The model under review builds one solid part; all positions refer to its coordinate system, in mm. A direction names the side the tool comes from. Round coordinates to 2 decimals unless told otherwise and drop trailing zeros. Write each loop counter-clockwise with the first axis right and the second up, starting at its lowest first coordinate (ties: lowest second). Pieces come first, ordered by that corner, then holes.
Item 1: Clearance check with flat-ended pins moving along their axes: pin 1 Ø5 at (y, z) = (-52, -5) entering from -X; pin 2 Ø8 at (x, y) = (-6.5, 62) entering from -Z; pin 3 Ø3 at (x, y) = (-4.5, 1) entering from +Z. State where each tip first meets the part, or that it passes through.
Item 2: Add section A-A (x = 0). Give the boundary of the cut face in (y, z) (3 decimals).
Item 3: Add section D-D (y = -61.5). Give the boundary of the cut face in (x, z) (3 decimals).
Item 4: Add section B-B (z = 0). Give the boundary of the cut face in (x, y) (3 decimals).
Item 5: Draft analysis for pull direction X (two halves, no side actions). For faces 1 (the face through (-7.559, -1.378, -5.796)), 2 (the face through (0, -66.675, 0)), 3 (the face through (0, 66.675, 0)), 4 (the face through (4, 98.425, -4)), state which applies: +X half, -X half, draft (parallel to the pull), parting line (faces both ways), or undercut.
Item 6: Add section C-C (y = 75.5). Give the boundary of the cut face in (x, z) (3 decimals), plus the area to 3 significant figures.
Item 7: Machinability: for faces 5 (the face through (0, -98.425, -6)), 6 (the face through (5.49, -82.77, 1.73)), 7 (the face through (-4.73, 82.77, 1.49)), which of the approach directions +Z, -Z, +X, -X, +Y, -Y give a long, thin tool a straight path to every point of the face, cutting with its end or side? Answer none if there is none.
Item 8: To check wall thickness, follow L1, parallel to Z at x = -0.25, y = 71; L2, parallel to Z at x = 0, y = -77 (3 decimals); L3, parallel to Y at x = 4.25, z = 3.25 (3 decimals). State the ranges of each line that lie inside material, in increasing order.
```python
from build123d import *

# Parameters (mm, degrees)
F0_R     = 9.525
F1_DEPTH = 98.425
F2_R     = 5.754688
F3_DEPTH = 31.75
F4_R     = 4.960938
F5_DEPTH = 31.75


with BuildPart() as f1:
    # F0 (on Front) → F1 (new body, symmetric)
    with BuildSketch(Plane.XZ):
        Circle(F0_R)
    extrude(amount=F1_DEPTH, both=True)

    # F2 (on face) → F3 (cut)
    with BuildSketch(Plane.XZ.offset(98.425)):
        Circle(F2_R)
    extrude(amount=-F3_DEPTH, mode=Mode.SUBTRACT)

    # F4 (on face) → F5 (cut)
    with BuildSketch(Plane(origin=(0, 98.425, 0), x_dir=(-1, 0, 0), z_dir=(0, 1, 0))):
        Circle(F4_R)
    extrude(amount=-F5_DEPTH, mode=Mode.SUBTRACT)


solid = f1.part
```
Numbers:
1. pin 1: stops at x = -9.19
1. pin 2: stops at z = -9.19
1. pin 3: stops at z = 9.04
2. outline: (-98.425, -9.525) - (98.425, -9.525) - (98.425, -4.961) - (66.675, -4.961) - (66.675, 4.961) - (98.425, 4.961) - (98.425, 9.525) - (-98.425, 9.525) - (-98.425, 5.755) - (-66.675, 5.755) - (-66.675, -5.755) - (-98.425, -5.755) - close
3. outline: circle Ø19.05 at (0, 0)
4. outline: (-9.525, -98.425) - (-5.755, -98.425) - (-5.755, -66.675) - (5.755, -66.675) - (5.755, -98.425) - (9.525, -98.425) - (9.525, 98.425) - (4.961, 98.425) - (4.961, 66.675) - (-4.961, 66.675) - (-4.961, 98.425) - (-9.525, 98.425) - close
5. face 1: parting line
5. face 2: undercut
5. face 3: undercut
5. face 4: draft
6. outline: circle Ø19.05 at (0, 0); hole circle Ø9.922 at (0, 0)
6. area: 208 mm2
7. face 5: +Z, -Z, +X, -X, -Y
7. face 6: -Y
7. face 7: +Y
8. L1: z = -9.52 to -4.95, 4.95 to 9.52
8. L2: z = -9.525 to -5.755, 5.755 to 9.525
8. L3: y = -66.675 to 98.425
